The listing builds one solid part. Answer for the finished solid, in the listing's coordinates (mm). A direction names the side the tool comes from. Give positions to 0.01 mm unless a question says otherwise; leave off trailing zeros. Order: outer loops, then holes, each group sorted by start corner. A loop starts at its lowest first (then second) coordinate and runs counter-clockwise, first axis right, second up. Notation, with made-up numbers: (8.5, 81) - (52.5, 81) arc R22 cw to (52.5, 100) - close; hole circle Ø2 at (-21, 37). An arc over 180 degrees is marked (long way). Answer as a JSON object with one key per item and string values. Group by question number.
Q1. Given pin 1 (3 mm diameter, centred on x = 1.5, y = 11.5, fed in from +Z); pin 2 (1 mm diameter, centred on y = 18, z = -1.5, fed in from -X); pin 3 (1.3 mm diameter, centred on x = 0, z = -0.5, fed in from +Y), each flat-ended and moving along its own axis, determine where each tip first touches the part or whether it passes through.
Q2. The mould has two halves that part along Z. Classify faces 1 (the face through (-1.88, 23.52, -1.07)), 2 (the face through (2, 15, 2)), 3 (the face through (-1.08, 19.19, -4.88)): released by +Z, released by -Z, zero draft, split by the parting line, or undercut.
Q3. A cutting plane is placed at C-C, the plane y = 8. Give the vertices of the cut face in (x, z), and give its area (3 significant figures).
Q4. A cutting plane is placed at B-B, the plane y = 19. Give the vertices of the cut face in (x, z), and give its area (3 significant figures).
Q5. For faces 4 (the face through (2.3, 25, 0.7)), 5 (the face through (0.54, 7.4, 2.44)), 6 (the face through (1.866, 23.521, -1.098)), determine the directions among +Z, -Z, +X, -X, +Y, -Y from which every point of the face is accessible in a straight line to the end or side of a thin tool.
Q6. Consider line 1 (Y direction, x = -0.75, z = -1.25); line 2 (Y direction, x = -1.5, z = -3.25); line 3 (Z direction, x = 1.75, y = 14.25). Determine where each line is inside the solid, lowest interval first.
Q7. A cutting plane is placed at A-A, the plane x = 0. Give the vertices of the cut face in (y, z), and give its area (3 significant figures).
Autodesk Inventor part; units mm, degrees
ref_plane "YZ Plane" through (0, 0, 0) normal (1, 0, 0) x (0, 1, 0)
ref_plane "XZ Plane" through (0, 0, 0) normal (0, 1, 0) x (-1, 0, 0)
ref_plane "XY Plane" through (0, 0, 0) normal (0, 0, 1) x (1, 0, 0)
sketch "Sketch1" plane through (0, 0, 0) normal (0, 1, 0) x (-1, 0, 0)
  circle A0 centre (0, 0) radius 2.5
  dimension "d0" = 5
extrude "Extrusion1" add sketch "Sketch1" along normal blind 15
sketch "Sketch2" plane through (0, 15, 0) normal (0, 1, 0) x (1, 0, 0)
  circle A0 centre (0, 0) radius 5
extrude "Extrusion2" add sketch "Sketch2" along normal blind 10
sketch "Sketch3" plane through (0, 25, 0) normal (0, 1, 0) x (1, 0, 0)
  circle A0 centre (0, 0) radius 2.5
  line L0 (2.5, 0) -> (1.25, -2.1651)
  line L1 (1.25, -2.1651) -> (-1.25, -2.1651)
  line L2 (-1.25, -2.1651) -> (-2.5, 0)
  line L3 (-2.5, 0) -> (-1.25, 2.1651)
  line L4 (-1.25, 2.1651) -> (1.25, 2.1651)
  line L5 (1.25, 2.1651) -> (2.5, 0)
fillet "Fillet1" radius 1.5 1 edges at (-5, 25, 0)
extrude "Extrusion3" cut sketch "Sketch3" against normal blind 3 contours L0 L1 L2 L3 L4 L5
properties part number "35mm_bolt"
Reply:
{
 "1": {"pin 1": "stops at z = 2.5", "pin 2": "stops at x = -4.9", "pin 3": "stops at y = 22"},
 "2": {"face 1": "undercut", "face 2": "zero draft", "face 3": "split by the parting line"},
 "3": {"outline": "circle Ø5 at (0, 0)", "area": "19.6 mm^2"},
 "4": {"outline": "circle Ø10 at (0, 0)", "area": "78.5 mm^2"},
 "5": {"face 4": "+Z, -Z, +X, -X, +Y", "face 5": "-Y", "face 6": "+Y"},
 "6": {"line 1": "y = 0 to 22", "line 2": "y = 15 to 25", "line 3": "z = -1.79 to 1.79"},
 "7": {"outline": "(0, -2.5) - (15, -2.5) - (15, -5) - (23.5, -5) arc R1.5 ccw to (25, -3.5) - (25, -2.17) - (22, -2.17) - (22, 2.17) - (25, 2.17) - (25, 3.5) arc R1.5 ccw to (23.5, 5) - (15, 5) - (15, 2.5) - (0, 2.5) - close", "area": "161 mm^2"}
}
